```python
from build123d import *

# Parameters (mm, degrees)
F1_DEPTH = 10


# Not quite as in the source:
# - a feature names something its author has since deleted; it is built from what else it names


with BuildPart() as f1:
    # F0 (on Top) → F1 (new body)
    with BuildSketch(Plane.XY):
        Polygon((-135, 145.3171813515), (-135, -111.8657903795), (-105, -111.8657903795), (-105, 115.3171813515), (0, 115.3171813515), (0, 145.3171813515), align=None)
        Polygon((81.1492523154, -181.6828186485), (81.1492523154, -211.6828186485), (135, -211.6828186485), (135, -33.1828186485), (105, -33.1828186485), (105, -181.6828186485), align=None)
        Polygon((105, -33.1828186485), (135, -33.1828186485), (135, 145.3171813515), (0, 145.3171813515), (0, 115.3171813515), (105, 115.3171813515), (105, -20.8807700001), align=None)
        Polygon((-135, -111.8657903795), (-135, -211.6828186485), (81.1492523154, -211.6828186485), (81.1492523154, -181.6828186485), (-105, -181.6828186485), (-105, -111.8657903795), align=None)
        Polygon((-105, -181.6828186485), (81.1492523154, -181.6828186485), (105, -181.6828186485), (105, -33.1828186485), (105, -20.8807700001), (105, 115.3171813515), (0, 115.3171813515), (-105, 115.3171813515), (-105, -111.8657903795), align=None)
        Polygon((-77.2907613296, 11.4150706229), (-77.2907613296, -33.1828186485), (-88.7750437384, -33.1828186485), (-88.7750437384, 11.4150706229), (-103.4829843671, 11.4150706229), (-103.4829843671, 20.9675284366), (-62.5946723856, 20.9675284366), (-62.5946723856, 11.4150706229), align=None, mode=Mode.SUBTRACT)
        with BuildLine():
            add(Edge.make_bspline(
                [(-39.1698177098, 6.8699495664), (-35.892826909, 8.9973269579), (-32.0410294035, 8.9973269579)],
                knots=[0, 0, 0, 1, 1, 1], degree=2))
            add(Edge.make_bspline(
                [(-32.0410294035, 8.9973269579), (-29.7418025848, 8.9973269579), (-28.2247869519, 8.6654797882)],
                knots=[0, 0, 0, 1, 1, 1], degree=2))
            Line((-28.2247869519, 8.6654797882), (-29.0781082454, -1.9180745884))
            add(Edge.make_bspline(
                [(-29.0781082454, -1.9180745884), (-30.4529036627, -1.5506723648), (-32.4084316271, -1.5506723648)],
                knots=[0, 0, 0, 1, 1, 1], degree=2))
            add(Edge.make_bspline(
                [(-32.4084316271, -1.5506723648), (-37.8127998194, -1.5506723648), (-40.8349794006, -4.3298924111)],
                knots=[0, 0, 0, 1, 1, 1], degree=2))
            add(Edge.make_bspline(
                [(-40.8349794006, -4.3298924111), (-43.8571589819, -7.1091124574), (-43.8571589819, -12.1105233722)],
                knots=[0, 0, 0, 1, 1, 1], degree=2))
            Line((-43.8571589819, -12.1105233722), (-43.8571589819, -33.1828186485))
            Line((-43.8571589819, -33.1828186485), (-55.1518144365, -33.1828186485))
            Line((-55.1518144365, -33.1828186485), (-55.1518144365, 8.2269674568))
            Line((-55.1518144365, 8.2269674568), (-46.5948981319, 8.2269674568))
            Line((-46.5948981319, 8.2269674568), (-44.9238105988, 1.258176893))
            Line((-44.9238105988, 1.258176893), (-44.3786331057, 1.258176893))
            add(Edge.make_bspline(
                [(-44.3786331057, 1.258176893), (-42.4468085106, 4.7425721749), (-39.1698177098, 6.8699495664)],
                knots=[0, 0, 0, 1, 1, 1], degree=2))
        make_face(mode=Mode.SUBTRACT)
        with BuildLine():
            add(Edge.make_bspline(
                [(14.4768327784, -1.0351240833), (16.9182798126, -5.8883889403), (16.9182798126, -12.406815488)],
                knots=[0, 0, 0, 1, 1, 1], degree=2))
            add(Edge.make_bspline(
                [(16.9182798126, -12.406815488), (16.9182798126, -22.5163024794), (11.5850217281, -28.2228886299)],
                knots=[0, 0, 0, 1, 1, 1], degree=2))
            add(Edge.make_bspline(
                [(11.5850217281, -28.2228886299), (6.2517636435, -33.9294747803), (-3.2651391162, -33.9294747803)],
                knots=[0, 0, 0, 1, 1, 1], degree=2))
            add(Edge.make_bspline(
                [(-3.2651391162, -33.9294747803), (-9.2265364863, -33.9294747803), (-13.7835092274, -31.3161783189)],
                knots=[0, 0, 0, 1, 1, 1], degree=2))
            add(Edge.make_bspline(
                [(-13.7835092274, -31.3161783189), (-18.3404819685, -28.7028818575), (-20.7819290028, -23.8140619466)],
                knots=[0, 0, 0, 1, 1, 1], degree=2))
            add(Edge.make_bspline(
                [(-20.7819290028, -23.8140619466), (-23.223376037, -18.9252420358), (-23.223376037, -12.406815488)],
                knots=[0, 0, 0, 1, 1, 1], degree=2))
            add(Edge.make_bspline(
                [(-23.223376037, -12.406815488), (-23.223376037, -2.2617734428), (-17.9315988487, 3.3677767576)],
                knots=[0, 0, 0, 1, 1, 1], degree=2))
            add(Edge.make_bspline(
                [(-17.9315988487, 3.3677767576), (-12.6398216604, 8.9973269579), (-3.0399571082, 8.9973269579)],
                knots=[0, 0, 0, 1, 1, 1], degree=2))
            add(Edge.make_bspline(
                [(-3.0399571082, 8.9973269579), (2.9214402619, 8.9973269579), (7.478413003, 6.4077338658)],
                knots=[0, 0, 0, 1, 1, 1], degree=2))
            add(Edge.make_bspline(
                [(7.478413003, 6.4077338658), (12.0353857441, 3.8181407736), (14.4768327784, -1.0351240833)],
                knots=[0, 0, 0, 1, 1, 1], degree=2))
        make_face(mode=Mode.SUBTRACT)
        with BuildLine():
            Line((64.2539082341, -33.1828186485), (55.5903267679, -33.1828186485))
            Line((55.5903267679, -33.1828186485), (54.0733111349, -27.8851156178))
            Line((54.0733111349, -27.8851156178), (53.4807269033, -27.8851156178))
            add(Edge.make_bspline(
                [(53.4807269033, -27.8851156178), (51.6674191546, -30.7769266681), (48.3311699306, -32.3532007242)],
                knots=[0, 0, 0, 1, 1, 1], degree=2))
            add(Edge.make_bspline(
                [(48.3311699306, -32.3532007242), (44.9949207066, -33.9294747803), (40.7401659236, -33.9294747803)],
                knots=[0, 0, 0, 1, 1, 1], degree=2))
            add(Edge.make_bspline(
                [(40.7401659236, -33.9294747803), (33.4395281901, -33.9294747803), (29.7358767425, -30.0184188517)],
                knots=[0, 0, 0, 1, 1, 1], degree=2))
            add(Edge.make_bspline(
                [(29.7358767425, -30.0184188517), (26.0322252949, -26.107362923), (26.0322252949, -18.7711701356)],
                knots=[0, 0, 0, 1, 1, 1], degree=2))
            Line((26.0322252949, -18.7711701356), (26.0322252949, 8.2269674568))
            Line((26.0322252949, 8.2269674568), (37.3268807495, 8.2269674568))
            Line((37.3268807495, 8.2269674568), (37.3268807495, -15.9623208777))
            add(Edge.make_bspline(
                [(37.3268807495, -15.9623208777), (37.3268807495, -20.4422576688), (38.9209323325, -22.6822260643)],
                knots=[0, 0, 0, 1, 1, 1], degree=2))
            add(Edge.make_bspline(
                [(38.9209323325, -22.6822260643), (40.5149839156, -24.9221944598), (43.9993791975, -24.9221944598)],
                knots=[0, 0, 0, 1, 1, 1], degree=2))
            add(Edge.make_bspline(
                [(43.9993791975, -24.9221944598), (48.7400530504, -24.9221944598), (50.8496529149, -21.7577946629)],
                knots=[0, 0, 0, 1, 1, 1], degree=2))
            add(Edge.make_bspline(
                [(50.8496529149, -21.7577946629), (52.9592527795, -18.5933948661), (52.9592527795, -11.2572020787)],
                knots=[0, 0, 0, 1, 1, 1], degree=2))
            Line((52.9592527795, -11.2572020787), (52.9592527795, 8.2269674568))
            Line((52.9592527795, 8.2269674568), (64.2539082341, 8.2269674568))
            Line((64.2539082341, 8.2269674568), (64.2539082341, -33.1828186485))
        make_face(mode=Mode.SUBTRACT)
        with BuildLine():
            add(Edge.make_bspline(
                [(103.9214966985, -15.5889928118), (105, -17.8111836804), (105, -20.8807700001)],
                knots=[0, 0, 0, 1, 1, 1], degree=2))
            add(Edge.make_bspline(
                [(105, -20.8807700001), (105, -27.2569763323), (100.5733957898, -30.5932255563)],
                knots=[0, 0, 0, 1, 1, 1], degree=2))
            add(Edge.make_bspline(
                [(100.5733957898, -30.5932255563), (96.1467915797, -33.9294747803), (87.3291382132, -33.9294747803)],
                knots=[0, 0, 0, 1, 1, 1], degree=2))
            add(Edge.make_bspline(
                [(87.3291382132, -33.9294747803), (82.8136463683, -33.9294747803), (79.6255432022, -33.3131871794)],
                knots=[0, 0, 0, 1, 1, 1], degree=2))
            add(Edge.make_bspline(
                [(79.6255432022, -33.3131871794), (76.4374400361, -32.6968995786), (73.6641458322, -31.5117311153)],
                knots=[0, 0, 0, 1, 1, 1], degree=2))
            Line((73.6641458322, -31.5117311153), (73.6641458322, -22.1844553097))
            add(Edge.make_bspline(
                [(73.6641458322, -22.1844553097), (76.8048422597, -23.6659158887), (80.7514532423, -24.6673832402)],
                knots=[0, 0, 0, 1, 1, 1], degree=2))
            add(Edge.make_bspline(
                [(80.7514532423, -24.6673832402), (84.6980642248, -25.6688505916), (87.6965404368, -25.6688505916)],
                knots=[0, 0, 0, 1, 1, 1], degree=2))
            add(Edge.make_bspline(
                [(87.6965404368, -25.6688505916), (93.847564761, -25.6688505916), (93.847564761, -22.1133452019)],
                knots=[0, 0, 0, 1, 1, 1], degree=2))
            add(Edge.make_bspline(
                [(93.847564761, -22.1133452019), (93.847564761, -20.7741048385), (93.0297985214, -19.9385610719)],
                knots=[0, 0, 0, 1, 1, 1], degree=2))
            add(Edge.make_bspline(
                [(93.0297985214, -19.9385610719), (92.2120322817, -19.1030173053), (90.2150234212, -18.048217373)],
                knots=[0, 0, 0, 1, 1, 1], degree=2))
            add(Edge.make_bspline(
                [(90.2150234212, -18.048217373), (88.2180145606, -16.9934174408), (84.887691179, -15.5949186541)],
                knots=[0, 0, 0, 1, 1, 1], degree=2))
            add(Edge.make_bspline(
                [(84.887691179, -15.5949186541), (80.1114622721, -13.5919839513), (77.8655680343, -11.8853413642)],
                knots=[0, 0, 0, 1, 1, 1], degree=2))
            add(Edge.make_bspline(
                [(77.8655680343, -11.8853413642), (75.6196737965, -10.1786987772), (74.6063547604, -7.9742854356)],
                knots=[0, 0, 0, 1, 1, 1], degree=2))
            add(Edge.make_bspline(
                [(74.6063547604, -7.9742854356), (73.5930357244, -5.7698720939), (73.5930357244, -2.5580655586)],
                knots=[0, 0, 0, 1, 1, 1], degree=2))
            add(Edge.make_bspline(
                [(73.5930357244, -2.5580655586), (73.5930357244, 2.9648194801), (77.8655680343, 5.981073219)],
                knots=[0, 0, 0, 1, 1, 1], degree=2))
            add(Edge.make_bspline(
                [(77.8655680343, 5.981073219), (82.1381003443, 8.9973269579), (89.9957672555, 8.9973269579)],
                knots=[0, 0, 0, 1, 1, 1], degree=2))
            add(Edge.make_bspline(
                [(89.9957672555, 8.9973269579), (97.4741802585, 8.9973269579), (104.549635984, 5.738113684)],
                knots=[0, 0, 0, 1, 1, 1], degree=2))
            Line((104.549635984, 5.738113684), (101.1482024945, -2.4039936584))
            add(Edge.make_bspline(
                [(101.1482024945, -2.4039936584), (98.0312094362, -1.0766049796), (95.32902534, -0.223283686)],
                knots=[0, 0, 0, 1, 1, 1], degree=2))
            add(Edge.make_bspline(
                [(95.32902534, -0.223283686), (92.6268412439, 0.6300376075), (89.8061403014, 0.6300376075)],
                knots=[0, 0, 0, 1, 1, 1], degree=2))
            add(Edge.make_bspline(
                [(89.8061403014, 0.6300376075), (84.8047293865, 0.6300376075), (84.8047293865, -2.0721464887)],
                knots=[0, 0, 0, 1, 1, 1], degree=2))
            add(Edge.make_bspline(
                [(84.8047293865, -2.0721464887), (84.8047293865, -3.5891621216), (86.4165584965, -4.703220477)],
                knots=[0, 0, 0, 1, 1, 1], degree=2))
            add(Edge.make_bspline(
                [(86.4165584965, -4.703220477), (88.0283876065, -5.8172788325), (93.4801625374, -7.9979888048)],
                knots=[0, 0, 0, 1, 1, 1], degree=2))
            add(Edge.make_bspline(
                [(93.4801625374, -7.9979888048), (98.327501552, -9.9653684538), (100.5852474745, -11.6660851985)],
                knots=[0, 0, 0, 1, 1, 1], degree=2))
            add(Edge.make_bspline(
                [(100.5852474745, -11.6660851985), (102.8429933969, -13.3668019433), (103.9214966985, -15.5889928118)],
                knots=[0, 0, 0, 1, 1, 1], degree=2))
        make_face(mode=Mode.SUBTRACT)
    extrude(amount=F1_DEPTH)


solid = f1.part
```
Geometry check sheet. Reference: the model listing, model coordinates, mm. A direction names the side the tool comes from. Give positions to 0.01 mm unless a question says otherwise; leave off trailing zeros. Write item = value, one per line. Start each with the question number.
1) Section check A-A (z = 3.5). Count the separate pieces of the cut face and the enclosed holes in it, then the cut area to 3 significant figures.
2) Scan lines: L1, parallel to Y at x = 91, z = 6; L2, parallel to Y at x = 3, z = 9.25; L3, parallel to Y at x = -32, z = 2.75. Record each from-to range of solid material in increasing order.
3) Access from +Z, -Z, +X, -X, +Y, -Y to the whole of each face (thin tool, end or side, straight path). Record for faces 5 (the flat face through (-96, 11.415, 5)), 6 (the flat face through (-135, -31, 5)).
4) Draft check along X on faces 1 (the flat face through (-43.857, -22, 5)), 2 (the flat face through (73.664, -27, 5)), 3 (the flat face through (135, -36, 5)), 4 (the flat face through (-2, -211.683, 5)). Enter one of: released by +X, released by -X, zero draft, split by the parting line, or undercut.
Geometry check:
q1.separate_pieces = 1
q1.enclosed_holes = 5
q1.area = 91,600 mm2
q2.L1 = -211.68 to -33.77, -25.31 to -18.48, -6.98 to 0.59, 8.98 to 145.32
q2.L2 = -211.68 to -33.2, 8.24 to 145.32
q2.L3 = -211.68 to -1.55, 9 to 145.32
q3.face_5 = +Z, -Z
q3.face_6 = +Z, -Z, -X, +Y, -Y
q4.face_1 = undercut
q4.face_2 = undercut
q4.face_3 = released by +X
q4.face_4 = zero draft
